For this review, take the finished solid that the model builds, in its own axes (mm). A direction names the side the tool comes from. Give positions to 0.01 mm unless a question says otherwise; leave off trailing zeros. Loops run counter-clockwise (first coordinate to the right, second up) from the corner with the lowest first, then second, coordinate; pieces in that order, holes last. Notation, with made-up numbers: (4, 71.5) -> (43, 71.5) arc R11 ccw to (43, 78.5) -> close; hole circle Ø7 at (-25, -8.75). An arc over 180 degrees is marked (long way). Write each question's results on one line, items separated by ' | '. Start each with the question number.
```python
from build123d import *

# Parameters (mm, degrees)
F0_W     = 200
F0_H     = 40
F0_R     = 50
F1_DEPTH = 20
F2_W     = 200
F2_H     = 40
F3_DEPTH = 200


with BuildPart() as f1:
    # F0 (on Front) → F1 (new body, symmetric)
    with BuildSketch(Plane.XZ):
        with Locations((0, 20)):
            Rectangle(F0_W, F0_H)
        with BuildLine():
            Line((-100, 200), (-100, 40))
            Line((-100, 40), (100, 40))
            Line((100, 40), (100, 200))
            ThreePointArc((100, 200), (0, 300), (-100, 200))
        make_face()
        with Locations((0, 200)):
            Circle(F0_R, mode=Mode.SUBTRACT)
    extrude(amount=F1_DEPTH, both=True)

    # F2 (on face) → F3 (join)
    with BuildSketch(Plane.XZ.offset(20)):
        with Locations((0, 20)):
            Rectangle(F2_W, F2_H)
    extrude(amount=F3_DEPTH)


solid = f1.part
```
1. Draft analysis for pull direction Z (two halves, no side actions). For faces 1 (the flat face through (-1, -98, 0)), 2 (the flat face through (-1, -220, 20)), 3 (the cylindrical face through (-10.84, 0.28, 151.19)), state which applies: released by +Z, released by -Z, zero draft, split by the parting line, or undercut.
2. We need section A-A (x = 0). Write out the cut boundary in (y, z), plus the area to 3 significant figures.
3. We need section D-D (x = -36.5). Write out the cut boundary in (y, z).
4. Machinability: for faces 4 (the flat face through (-1, 20, 119)), 5 (the flat face through (-1, -20, 143)), which of the approach directions +Z, -Z, +X, -X, +Y, -Y give a long, thin tool a straight path to every point of the face, cutting with its end or side? Answer none if there is none.
5. Wall thickness on L1, parallel to Z at x = 0, y = -11; L2, parallel to Z at x = -90.5, y = -67; L3, parallel to Y at x = 58.5, z = 90: over which ranges is each line inside the solid? List them lowest first.
6. We need section C-C (y = 1). Write out the cut boundary in (x, z), plus the area to 3 significant figures.
7. For pin 1 Ø4 at (x, y) = (51, -118) entering from +Z; pin 2 Ø8 at (x, z) = (-64, 49.5) entering from -Y, all flat-tipped, find the tip position at first contact; note any pin that passes through.
8. We need section B-B (z = 168). Write out the cut boundary in (x, y), plus the area to 3 significant figures.
Response:
1) face 1: released by -Z | face 2: zero draft | face 3: undercut
2) outline: (-220, 0) -> (20, 0) -> (20, 150) -> (-20, 150) -> (-20, 40) -> (-220, 40) -> close; (-20, 250) -> (20, 250) -> (20, 300) -> (-20, 300) -> close | area: 16,000 mm2
3) outline: (-220, 0) -> (20, 0) -> (20, 165.83) -> (-20, 165.83) -> (-20, 40) -> (-220, 40) -> close; (-20, 234.17) -> (20, 234.17) -> (20, 293.1) -> (-20, 293.1) -> close
4) face 4: +Z, -Z, +X, -X, +Y | face 5: +Z, +X, -X, -Y
5) L1: z = 0 to 150, 250 to 300 | L2: z = 0 to 40 | L3: y = -20 to 20
6) outline: (-100, 0) -> (100, 0) -> (100, 200) arc R100 ccw to (-100, 200) -> close; hole circle Ø100 at (0, 200) | area: 47,900 mm2
7) pin 1: stops at z = 40 | pin 2: stops at y = -20
8) outline: (-100, -20) -> (-38.42, -20) -> (-38.42, 20) -> (-100, 20) -> close; (38.42, -20) -> (100, -20) -> (100, 20) -> (38.42, 20) -> close | area: 4,930 mm2
